For this review, use the dimensioned drawing (mm, ordinates from the lowest corner) and the shaded views. A direction names the side the tool comes from. Coordinates: 2 decimals unless noted, no trailing zeros. Order: outer loops, then holes, each group sorted by start corner. A loop starts at its lowest first (then second) coordinate and runs counter-clockwise, first axis right, second up. Notation, with made-up numbers: M -35.75,-19.5 L -0.75,-19.5 A20 cw -0.75,17.5 Z; hole C 88,-39 d9. An arc over 180 degrees is marked long. Answer in a Markdown table with one row per item.
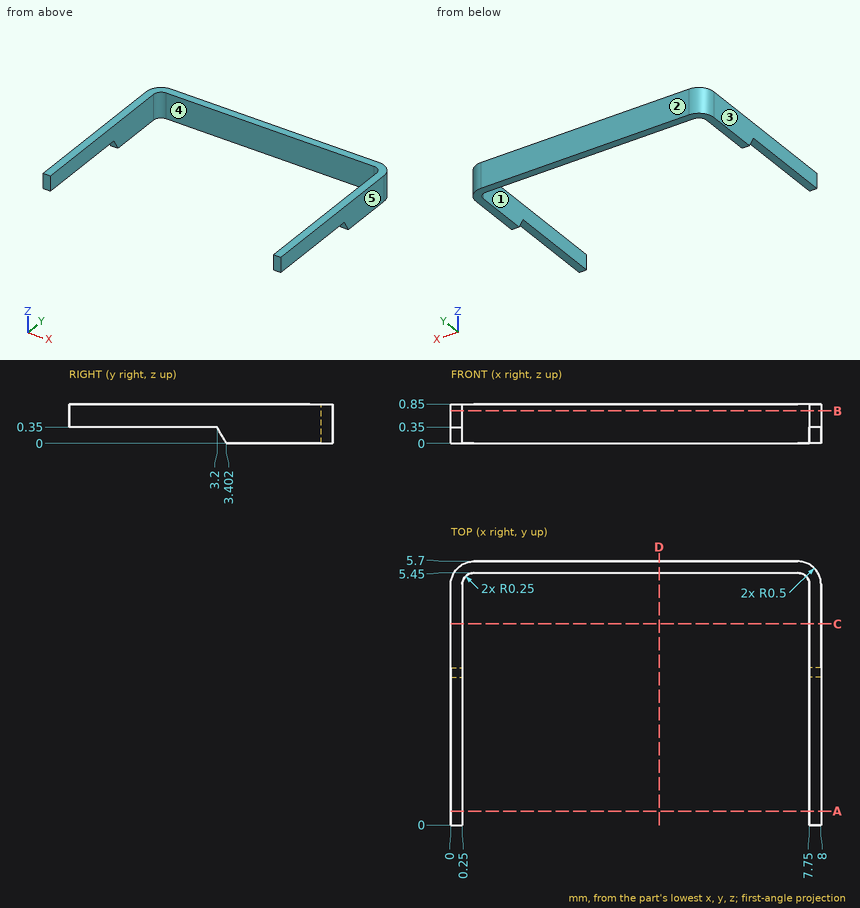
(1) Machinability: for the marked faces 1 and 2, which of the approach directions +Z, -Z, +X, -X, +Y, -Y give a long, thin tool a straight path to every point of the face, cutting with its end or side? Answer none if there is none.
Report:
| item | result |
|---|---|
| face 1 | +Z, -Z, -Y |
| face 2 | +Z, -Z, +X, -X, +Y |
(2) Take a section at D-D (x = 4.5). Write out the cut boundary in (y, z).
Report:
| item | result |
|---|---|
| outline | M 5.45,0 L 5.7,0 L 5.7,0.85 L 5.45,0.85 Z |
(3) Take a section at C-C (y = 4.35). Write out the cut boundary in (x, z).
Report:
| item | result |
|---|---|
| outline | M 0,0 L 0.25,0 L 0.25,0.85 L 0,0.85 Z; M 7.75,0 L 8,0 L 8,0.85 L 7.75,0.85 Z |
(4) Take a section at B-B (z = 0.7). Write out the cut boundary in (x, y).
Report:
| item | result |
|---|---|
| outline | M 0,0 L 0.25,0 L 0.25,5.2 A0.25 cw 0.5,5.45 L 7.5,5.45 A0.25 cw 7.75,5.2 L 7.75,0 L 8,0 L 8,5.2 A0.5 ccw 7.5,5.7 L 0.5,5.7 A0.5 ccw 0,5.2 Z |
(5) The part is to be moulded in two halves that separate along X. For the marked faces 3, 4 and 5, say which applies: +X half, -X half, draft (parallel to the pull), parting line (faces both ways), or undercut.
Report:
| item | result |
|---|---|
| face 3 | -X half |
| face 4 | undercut |
| face 5 | +X half |
(6) Take a section at A-A (y = 0.3). Write out the cut boundary in (x, z).
Report:
| item | result |
|---|---|
| outline | M 0,0.35 L 0.25,0.35 L 0.25,0.85 L 0,0.85 Z; M 7.75,0.35 L 8,0.35 L 8,0.85 L 7.75,0.85 Z |
(7) To check wall thickness, follow line 1 (X direction, y = 2.9, z = 0.7); line 2 (Y direction, x = 6, z = 0.4); line 3 (X direction, y = 5.3, z = 0.6). State the ranges of each line that lie inside material, in increasing order. Write a range as [from, to].
Report:
| item | result |
|---|---|
| line 1 | [0, 0.25], [7.75, 8] |
| line 2 | [5.45, 5.7] |
| line 3 | [0.01, 0.27], [7.73, 7.99] |
(8) Insertion check: P1, Ø1.5, axis at x = 1.5, y = 3, coming from the +Z side. The pin has a flat end and moves straight along its axis. Give the tip position at first contact, or say it passes through.
Report:
| item | result |
|---|---|
| P1 | through |
